Answer from the drawing. Dimensions are ordinates in mm from the lowest x, y and z of the part. A direction names the side the tool comes from. Give positions to 0.01 mm unless a question says otherwise; leave off trailing zeros. Write each loop counter-clockwise with the first axis right and the second up, starting at its lowest first coordinate (ties: lowest second). Pieces come first, ordered by that corner, then holes. Notation, with made-up numbers: M 8.5,-3.75 L 42.5,-3.75 A32 ccw 42.5,32.25 Z; hole C -36,32.25 d8. An arc over 180 degrees is marked long. Answer as a JSON object with one key per item and string values.
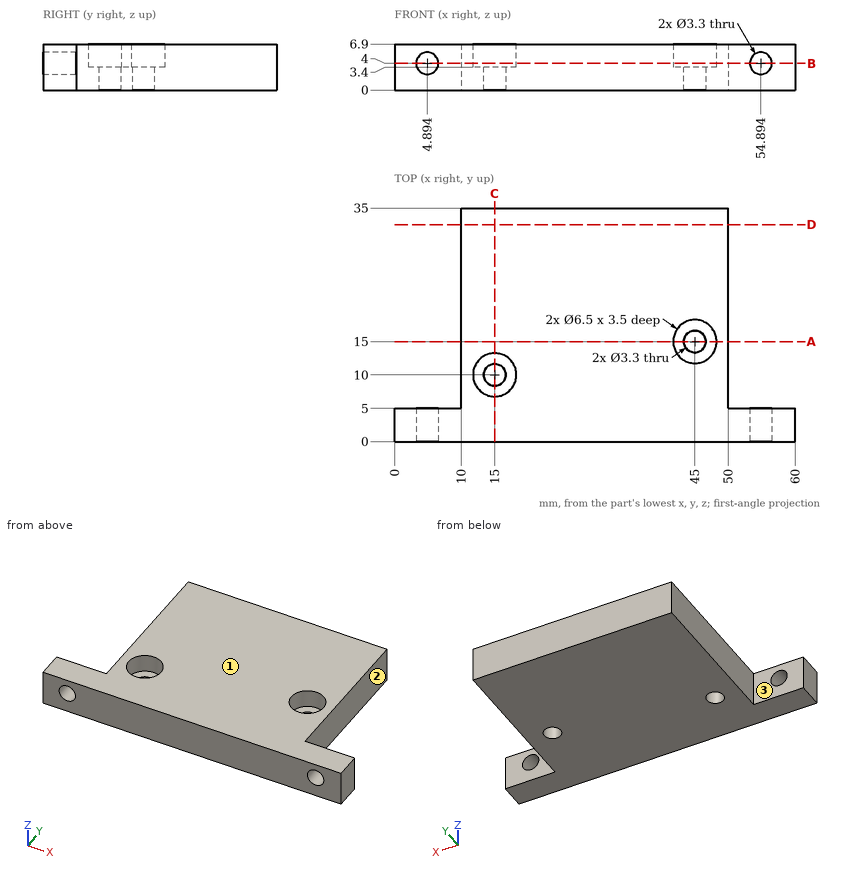
1. Consider line 1 along X through (y, z) = (3.85, 4); line 2 along X through (y, z) = (15, 1.6); line 3 along Y through (x, z) = (45, 1.15). Determine where each line is inside the solid, lowest interval first.
Verdict:
{"line 1": "x = 0 to 3.24, 6.54 to 53.24, 56.54 to 60", "line 2": "x = 10 to 43.35, 46.65 to 50", "line 3": "y = 0 to 13.35, 16.65 to 35"}
2. A cutting plane is placed at C-C, the plane x = 15. Give the vertices of the cut face in (y, z).
Verdict:
{"outline": "M 0,0 L 8.35,0 L 8.35,3.4 L 6.75,3.4 L 6.75,6.9 L 0,6.9 Z; M 11.65,0 L 35,0 L 35,6.9 L 13.25,6.9 L 13.25,3.4 L 11.65,3.4 Z"}
3. A cutting plane is placed at D-D, the plane y = 32.5. Give the vertices of the cut face in (x, z), plus the area to 3 significant figures.
Verdict:
{"outline": "M 10,0 L 50,0 L 50,6.9 L 10,6.9 Z", "area": "276 mm2"}
4. A cutting plane is placed at A-A, the plane y = 15. Give the vertices of the cut face in (x, z), plus the area to 3 significant figures.
Verdict:
{"outline": "M 10,0 L 43.35,0 L 43.35,3.4 L 41.75,3.4 L 41.75,6.9 L 10,6.9 Z; M 46.65,0 L 50,0 L 50,6.9 L 48.25,6.9 L 48.25,3.4 L 46.65,3.4 Z", "area": "242 mm2"}
5. A cutting plane is placed at B-B, the plane z = 4. Give the vertices of the cut face in (x, y).
Verdict:
{"outline": "M 0,0 L 3.24,0 L 3.24,5 L 0,5 Z; M 6.54,0 L 53.24,0 L 53.24,5 L 50,5 L 50,35 L 10,35 L 10,5 L 6.54,5 Z; M 56.54,0 L 60,0 L 60,5 L 56.54,5 Z; hole C 15,10 d6.5; hole C 45,15 d6.5"}
6. Flat-ended cylindrical pins translate along their axes: pin 1 (2.5 mm diameter, centred on x = 54.89, z = 4, fed in from +Y); pin 2 (1 mm diameter, centred on x = 8.5, z = 1.5, fed in from +Y); pin 3 (2 mm diameter, centred on y = 27, z = 4, fed in from +X); pin 4 (4 mm diameter, centred on y = 16, z = 5, fed in from -X). Find the tip coordinate at first contact, or state that the pin passes through.
Verdict:
{"pin 1": "passes through", "pin 2": "stops at y = 5", "pin 3": "stops at x = 50", "pin 4": "stops at x = 10"}
7. For the marked faces 1, 2 and 3, determine the directions among +Z, -Z, +X, -X, +Y, -Y from which every point of the face is accessible in a straight line to the end or side of a thin tool.
Verdict:
{"face 1": "+Z, +X, -X, +Y, -Y", "face 2": "+Z, -Z, +X, +Y", "face 3": "+Z, -Z, -X, +Y"}
